```python
from build123d import *

# Parameters (mm, degrees)
SKETCH_1_R      = 16
SKETCH_1_R_2    = 8
SKETCH_1_R_3    = 2.15
SKETCH_1_R_4    = 4
EXTRUDE_2_DEPTH = 3
SKETCH_2_R      = 8
SKETCH_2_R_2    = 4
EXTRUDE_3_DEPTH = 10


with BuildPart() as part:
    # 草图1 → 凸台-拉伸2 (new body)
    # profile 1 of 3: a face of its own
    with BuildSketch(Plane.XY):
        Circle(SKETCH_1_R)
        Circle(SKETCH_1_R_2, mode=Mode.SUBTRACT)
        with Locations((12, 0)):
            Circle(SKETCH_1_R_3, mode=Mode.SUBTRACT)
        with Locations((-12, 0)):
            Circle(SKETCH_1_R_3, mode=Mode.SUBTRACT)
        with Locations((0, -12)):
            Circle(SKETCH_1_R_3, mode=Mode.SUBTRACT)
        with Locations((0, 12)):
            Circle(SKETCH_1_R_3, mode=Mode.SUBTRACT)
    # profile 2 of 3: a face of its own
    with BuildSketch(Plane.XY):
        Circle(SKETCH_1_R_2)
        Circle(SKETCH_1_R_4, mode=Mode.SUBTRACT)
    # profile 3 of 3: a face of its own
    with BuildSketch(Plane.XY):
        Circle(SKETCH_1_R_4)
    extrude(amount=EXTRUDE_2_DEPTH)

    # 草图2 → 凸台-拉伸3 (add)
    with BuildSketch(Plane.XY.offset(3)):
        Circle(SKETCH_2_R)
        Circle(SKETCH_2_R_2, mode=Mode.SUBTRACT)
    extrude(amount=EXTRUDE_3_DEPTH)


solid = part.part
```
For this review, take the finished solid that the model builds, in its own axes (mm). A direction names the side the tool comes from. Coordinates: 2 decimals unless noted, no trailing zeros. Write each loop counter-clockwise with the first axis right and the second up, starting at its lowest first coordinate (ties: lowest second). Pieces come first, ordered by that corner, then holes.
(1) Add section B-B on y = -13. Give the boundary of the cut face in (x, z), then the cut area to 3 significant figures.
(2) Add section A-A on x = 0. Give the boundary of the cut face in (y, z), then the cut area to 3 significant figures.
(3) The part is to be moulded in two halves that separate along X. For faces 1 (the face through (-1.73, -7.81, 7.93)), 2 (the face through (14.05, 0.65, 1.48)), 3 (the face through (-4, -2, 13)), say which applies: +X half, -X half, draft (parallel to the pull), parting line (faces both ways), or undercut.
(4) For pin 1 Ø4 at (y, z) = (1.5, 7.5) entering from +X; pin 2 Ø7 at (x, y) = (0, 12) entering from +Z; pin 3 Ø5 at (x, z) = (-9.5, 5) entering from -Y; pin 4 Ø3.5 at (x, y) = (12, 0) entering from -Z (1 decimal), all flat-tipped, find the tip position at first contact; note any pin that passes through.
(5) Tool access review of faces 4 (the face through (-1.706, 10.692, 1.479)), 5 (the face through (0, 0, 3)): name each direction out of +Z, -Z, +X, -X, +Y, -Y from which nothing blocks a thin tool from reaching the whole face with its end or side.
(6) Add section C-C on z = 1.5. Give the boundary of the cut face in (x, y).
(7) Wall thickness on probe 1 along Y at (x, z) = (0, 1.1); probe 2 along Z at (x, y) = (4, 12); probe 3 along Y at (x, z) = (0.5, 9): over which ranges is each line inside the solid? List them lowest first.
Answer sheet:
1. outline: (-9.33, 0) - (-1.9, 0) - (-1.9, 3) - (-9.33, 3) - close; (1.9, 0) - (9.33, 0) - (9.33, 3) - (1.9, 3) - close
1. area: 44.5 mm2
2. outline: (-16, 0) - (-14.15, 0) - (-14.15, 3) - (-16, 3) - close; (-9.85, 0) - (9.85, 0) - (9.85, 3) - (8, 3) - (8, 13) - (4, 13) - (4, 3) - (-4, 3) - (-4, 13) - (-8, 13) - (-8, 3) - (-9.85, 3) - close; (14.15, 0) - (16, 0) - (16, 3) - (14.15, 3) - close
2. area: 150 mm2
3. face 1: parting line
3. face 2: undercut
3. face 3: draft
4. pin 1: stops at x = 8
4. pin 2: stops at z = 3
4. pin 3: stops at y = -13.86
4. pin 4: passes through
5. face 4: +Z, -Z
5. face 5: +Z
6. outline: circle Ø32 at (0, 0); hole circle Ø4.3 at (-12, 0); hole circle Ø4.3 at (0, -12); hole circle Ø4.3 at (0, 12); hole circle Ø4.3 at (12, 0)
7. probe 1: y = -16 to -14.15, -9.85 to 9.85, 14.15 to 16
7. probe 2: z = 0 to 3
7. probe 3: y = -7.98 to -3.97, 3.97 to 7.98
